```python
from build123d import *

# Parameters (mm, degrees)
F0_W     = 203.2
F0_H     = 247.65
F1_DEPTH = 19.05
F2_W     = 19.05
F2_H     = 12.7
F3_DEPTH = 203.201
F4_SIZE  = 19.04999
F5_SIZE  = 19.04999


# Not quite as in the source:
# - a fillet or chamfer is up to 0.001 mm smaller than in the source, because OpenCascade refuses the exact size


with BuildPart() as f1:
    # F0 (on Top) → F1 (new body)
    with BuildSketch(Plane.XY):
        Rectangle(F0_W, F0_H)
    extrude(amount=F1_DEPTH)

    # F2 (on face) → F3 (cut, through all)
    with BuildSketch(Plane(origin=(-101.6, 0, 0), x_dir=(0, -1, 0), z_dir=(-1, 0, 0))):
        with Locations((-114.3, 6.35)):
            Rectangle(F2_W, F2_H)
    extrude(amount=-F3_DEPTH, mode=Mode.SUBTRACT)

    # F4 (size 19.05 in the source; OpenCascade refuses exactly that, so slightly less here)
    f4_edges = [f1.edges().sort_by_distance(p)[0] for p in [
        (-101.6, -9.525, 0),
    ]]
    chamfer(f4_edges, length=F4_SIZE)

    # F5 (size 19.05 in the source; OpenCascade refuses exactly that, so slightly less here)
    f5_edges = [f1.edges().sort_by_distance(p)[0] for p in [
        (101.6, -9.525, 0),
    ]]
    chamfer(f5_edges, length=F5_SIZE)


solid = f1.part
```
Check sheet for the modelled part. Datum: model origin and axes. Units: mm. A direction names the side the tool comes from. Coordinates: 2 decimals unless noted, no trailing zeros. Write each loop counter-clockwise with the first axis right and the second up, starting at its lowest first coordinate (ties: lowest second). Pieces come first, ordered by that corner, then holes. Notation, with made-up numbers: M -15.5,15.25 L -3.5,15.25 A24 cw -3.5,40.25 Z; hole C 66.5,5.5 d9. An arc over 180 degrees is marked long. Write item = value, one per line. Start each with the question number.
1. Sectioned sample at C-C (z = 7). Record the cut outline in (x, y) (3 decimals).
2. Tool access check on faces 1 (the flat face through (-1, 114, 12.7)), 2 (the flat face through (-1, -8, 0)). Record the directions out of +Z, -Z, +X, -X, +Y, -Y that give a thin tool (end or side, any length) a straight path to the whole face; none if there is none.
3. Thickness scan on probe 1 along Y at (x, z) = (-79.5, 9.25) (3 decimals); probe 2 along X at (y, z) = (-14.5, 2.5); probe 3 along X at (y, z) = (-24, 14). Record the ranges inside material, lowest first.
4. Sectioned sample at A-A (x = 54.5). Record the cut outline in (y, z) (3 decimals).
5. Go/stop test with flat-tipped pins: pin 1 (10 mm diameter, centred on x = -6, z = 6, fed in from +Y) (3 decimals); pin 2 (21 mm diameter, centred on x = 11, y = 111, fed in from -Z); pin 3 (5 mm diameter, centred on y = 8, z = 12, fed in from +X); pin 4 (2 mm diameter, centred on y = 2, z = 9.5, fed in from -X). Record where each tip stops, or that it passes through.
The answers:
q1.outline = M -89.55,-123.825 L 89.55,-123.825 L 89.55,104.775 L -89.55,104.775 Z
q2.face_1 = -Z, +X, -X, +Y
q2.face_2 = -Z, +X, -X, +Y, -Y
q3.probe_1 = -123.825 to 104.775
q3.probe_2 = -85.05 to 85.05
q3.probe_3 = -96.55 to 96.55
q4.outline = M -123.825,0 L 104.775,0 L 104.775,12.7 L 123.825,12.7 L 123.825,19.05 L -123.825,19.05 Z
q5.pin_1 = 104.775
q5.pin_2 = 0
q5.pin_3 = 97.05
q5.pin_4 = -93.05
